Check sheet for the modelled part. Datum: model origin and axes. Units: mm. Face numbers are marked on the shaded views. Give positions to 0.01 mm unless a question says otherwise; leave off trailing zeros. Loops run counter-clockwise (first coordinate to the right, second up) from the corner with the lowest first, then second, coordinate; pieces in that order, holes last. Notation, with made-up numbers: M 66.5,21 L 125.5,21 A21 ccw 125.5,38 Z; hole C -39.5,29.25 d9. An arc over 180 degrees is marked long. Use one line per item in the form item = value.
from build123d import *

# Parameters (mm, degrees)
EXTRUDE_1_DEPTH     = 30
SKETCH_2_R          = 3
CUT_EXTRUDE_1_DEPTH = 192
FILLET_1_R          = 15
CUT_EXTRUDE_2_DEPTH = 192
SKETCH_4_R          = 3
EXTRUDE_2_DEPTH     = 66
FILLET_2_R          = 15
FILLET_3_R          = 15
FILLET_4_R          = 15
FILLET_5_R          = 15
FILLET_8_ANGLE      = 6.858136


with BuildPart() as part:
    # 草图1 → 凸台-拉伸1 (new body)
    with BuildSketch(Plane.XY):
        with BuildLine():
            Line((35, -93.674969976), (35, 93.674969976))
            ThreePointArc((35, 93.674969976), (0, 100), (-35, 93.674969976))
            Line((-35, 93.674969976), (-35, -93.674969976))
            ThreePointArc((-35, -93.674969976), (0, -100), (35, -93.674969976))
        make_face()
    extrude(amount=EXTRUDE_1_DEPTH)

    # 草图2 → 切除-拉伸1 (cut)
    with BuildSketch(Plane(origin=(35, 0, 0), x_dir=(0, 0, -1), z_dir=(1, 0, 0))):
        with Locations((-15, 83.674969976)):
            Circle(SKETCH_2_R)
    extrude(amount=-CUT_EXTRUDE_1_DEPTH, mode=Mode.SUBTRACT)

    # 圆角1
    fillet_1_edges = [part.edges().sort_by_distance(p)[0] for p in [
        (0, 100, 0),
    ]]
    fillet(fillet_1_edges, radius=FILLET_1_R)

    # 草图3 → 切除-拉伸2 (cut)
    with BuildSketch(Plane.XY.offset(30)):
        Polygon((0, -100), (-30, -100), (-30, 70), (30, 70), (30, -100), align=None)
    extrude(amount=-CUT_EXTRUDE_2_DEPTH, mode=Mode.SUBTRACT)

    # 草图4 → 凸台-拉伸2 (add)
    with BuildSketch(Plane(origin=(35, 0, 0), x_dir=(0, 0, -1), z_dir=(1, 0, 0))):
        with Locations((-15, -80.393920142)):
            Circle(SKETCH_4_R)
    extrude(amount=-EXTRUDE_2_DEPTH)

    # 圆角2
    fillet_2_edges = [part.edges().sort_by_distance(p)[0] for p in [
        (0, 100, 30),
    ]]
    fillet(fillet_2_edges, radius=FILLET_2_R - 0.0001)  # a hair under: the kernel refuses the full size

    # 圆角3
    # the kernel refuses this fillet: 15 mm, written as the material it takes off along each edge
    with BuildSketch(Plane(origin=(0, 0, 30), x_dir=(-0.07024960756428812, -0.9975294444962832, 0), z_dir=(-0.9975294444962832, 0.07024960756428812, 0))) as fillet_3_piece_1:
        with BuildLine():
            CenterArc((100 - FILLET_3_R, -FILLET_3_R), FILLET_3_R, 0, 90)
            Line((100, -FILLET_3_R), (100, 0))
            Line((100, 0), (100 - FILLET_3_R, 0))
        make_face()
    revolve(axis=Axis((0, 0, 30), (0, 0, 1)), revolution_arc=46.001566182, mode=Mode.SUBTRACT)

    # 圆角4
    # the kernel refuses this fillet: 15 mm, written as the material it takes off along each edge
    with BuildSketch(Plane(origin=(0, 0, 0), x_dir=(-0.07024960756429688, -0.9975294444962826, 0), z_dir=(-0.9975294444962826, 0.07024960756429688, 0))) as fillet_4_piece_1:
        with BuildLine():
            CenterArc((100 - FILLET_4_R, FILLET_4_R), FILLET_4_R, 270, 90)
            Line((100, FILLET_4_R), (100, 0))
            Line((100, 0), (100 - FILLET_4_R, 0))
        make_face()
    revolve(axis=Axis((0, 0, 0), (0, 0, 1)), revolution_arc=46.001566182, mode=Mode.SUBTRACT)

    # 圆角5
    # the kernel refuses this fillet: 15 mm, written as the material it takes off along each edge
    with BuildSketch(Plane(origin=(0, 0, 30), x_dir=(-0.668783476201052, -0.7434572361342896, 0), z_dir=(-0.7434572361342896, 0.668783476201052, 0))) as fillet_5_piece_1:
        with BuildLine():
            CenterArc((100 - FILLET_5_R, -FILLET_5_R), FILLET_5_R, 0, 90)
            Line((100 - FILLET_5_R, 0), (100, 0))
            Line((100, 0), (100, -FILLET_5_R))
        make_face()
    revolve(axis=Axis((0, 0, 30), (0, 0, 1)), revolution_arc=46.001566182, mode=Mode.SUBTRACT)

    # 圆角8: read off the stored shape, not the designer's step
    # 圆角8 outline → 圆角8 (revolve, cut)
    with BuildSketch(Plane(origin=(0, 0, 0), x_dir=(-0.4117647058823542, -0.911290199107627, 0), z_dir=(-0.911290199107627, 0.4117647058823542, 0))):
        with BuildLine():
            ThreePointArc((100, 15), (95.606601718, 4.393398282), (85, 0))
            Line((85, 0), (100, 0))
            Line((100, 0), (100, 15))
        make_face()
    revolve(axis=Axis((0, 0, 0), (0, 0, 1)), revolution_arc=FILLET_8_ANGLE, mode=Mode.SUBTRACT)


solid = part.part
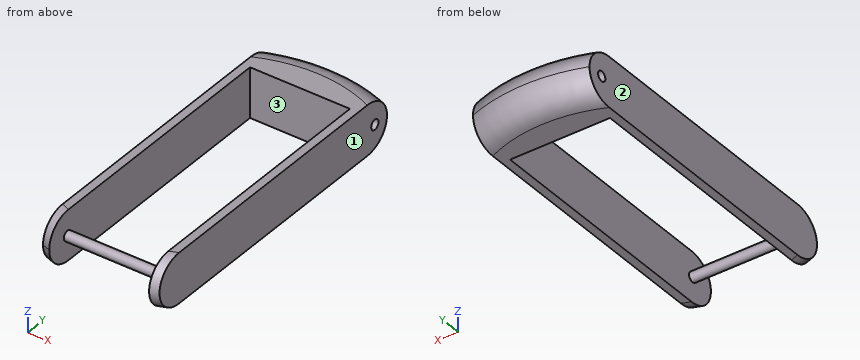
1) Scan lines: line 1 (Y direction, x = -2, z = 15); line 2 (X direction, y = 8, z = 11.5); line 3 (Y direction, x = 24, z = 12.5). Record each from-to range of solid material in increasing order.
Evaluation:
line_1 = -83.39 to -77.39, 70 to 80.67, 86.67 to 99.98
line_2 = -35 to -30, 30 to 35
line_3 = -82.05 to -78.74, 70 to 82.02, 85.33 to 96.86
2) Depth check by flat-ended pin: pin 1 Ø10 at (x, z) = (-13, 23.5) entering from -Y. Enter the tip coordinate at first touch or a pass-through.
Evaluation:
pin_1 = 70
3) Section check C-C (z = 7). Record the cut outline in (x, y), then the cut area to 3 significant figures.
Evaluation:
outline = M -35,-91.2 A97.69 ccw -30,-92.97 L -30,70 L 30,70 L 30,-92.97 A97.69 ccw 35,-91.2 L 35,91.2 A97.69 ccw -35,91.2 Z
area = 3,410 mm^2
4) Section check B-B (x = 25). State how many separate pieces and enclosed holes the cut face has, then the cut area to 3 significant figures.
Evaluation:
separate_pieces = 2
enclosed_holes = 1
area = 705 mm^2
5) Release check for a two-part mould opening along X. For the marked faces 1, 2 and 3 record: pulls with the +X half, pulls with the -X half, needs draft (parallel to the pull), parting line crosses it, or undercut.
Evaluation:
face_1 = pulls with the +X half
face_2 = pulls with the -X half
face_3 = undercut
6) Section check A-A (y = -15). Record the cut outline in (x, z), then the cut area to 3 significant figures.
Evaluation:
outline = M -35,0 L -30,0 L -30,30 L -35,30 Z; M 30,0 L 35,0 L 35,30 L 30,30 Z
area = 300 mm^2
